Build history of the part. All positions in model axes, mm. Face numbers are marked on the shaded views. A direction names the side the tool comes from. Round coordinates to 2 decimals unless told otherwise and drop trailing zeros. Use one line per item in the form item = value. Start each with the question number.
Q1. 3-axis set-ups, long thin cutter, end or side, ignore diameter. For the marked faces 1 and 2: which of +Z, -Z, +X, -X, +Y, -Y reach the whole face in a straight line?
Q2. Saw through at A-A (y = -77.5). Count the separate pieces of the cut face and the enclosed holes in it, then the cut area to 3 significant figures.
Q3. Drill centre lines: line 1 (X direction, y = -75.5, z = -2); line 2 (Z direction, x = -5.5, y = 35.5); line 3 (X direction, y = -37.5, z = 6.5). Where is each one in solid material? Low to high.
Q4. Pin check, flat tips, straight feed: pin 1 (13.5 mm diameter, centred on x = -6, y = 66, fed in from +Z); pin 2 (0.5 mm diameter, centred on x = 22, y = -31.5, fed in from -Z); pin 3 (1.6 mm diameter, centred on x = 0.5, z = 8, fed in from -Y). Stop position of each tip, or through.
```python
from build123d import *

# Parameters (mm, degrees)
F2_DEPTH       = 250
F3_W           = 38
F3_H           = 13
F4_DEPTH       = 250
F5_R           = 9
F6_R           = 1
F7_T1_DEPTH    = 509.3674969976
F9_DEPTH       = 500.001
F12_DEPTH      = 13.5192964571
F12_DEPTH_BACK = 10.001
F13_T1_DEPTH   = 2
F13_T6_DEPTH   = 16.7634354909
F13_S7_R       = 200
F13_T8_DEPTH   = 11
F13_T12_DEPTH  = 16.7632527384
F13_S13_R      = 200
F13_T14_DEPTH  = 11
F13_T15_DEPTH  = 29.2634354909
F13_T17_DEPTH  = 27
F13_T19_DEPTH  = 29.2632527384
F14_DEPTH      = 13.5192964571
F14_DEPTH_BACK = 10.001


# Not quite as in the source:
# - a fillet or chamfer that OpenCascade refuses, or shapes differently, is made with other operations: its cross-section is extruded or revolved along the edge and cut away or added


with BuildPart() as f2:
    # F0 (on Front) → F2 (new body, symmetric)
    with BuildSketch(Plane.XZ):
        with BuildLine():
            Line((-22.5004640741, 10), (-45.5824640741, 10))
            Line((-45.5824640741, 10), (-57.5, 0))
            Line((-57.5, 0), (-57.5, -4))
            Line((-57.5, -4), (-40.1794919243, -14))
            ThreePointArc((-40.1794919243, -14), (0.0006744682, -9.9223168214), (40.1808408606, -14))
            Line((40.1808408606, -14), (57.5, -4.0007788087))
            Line((57.5, -4.0007788087), (57.5, -0.0007788087))
            Line((57.5, -0.0007788087), (45.5815359259, 10))
            Line((45.5815359259, 10), (22.4995359259, 10))
            Line((22.4995359259, 10), (22.4995359259, 8.7))
            Line((22.4995359259, 8.7), (-22.5004640741, 8.7))
            Line((-22.5004640741, 8.7), (-22.5004640741, 10))
        make_face()
    extrude(amount=F2_DEPTH, both=True)

    # F3 (on Front) → F4 (cut, symmetric)
    with BuildSketch(Plane.XZ):
        with Locations((0, 0.2)):
            Rectangle(F3_W, F3_H)
    extrude(amount=F4_DEPTH, both=True, mode=Mode.SUBTRACT)

    # F5
    f5_edges = [f2.edges().sort_by_distance(p)[0] for p in [
        (45.581536, 0, 10),
        (40.180841, 0, -14),
        (-45.582464, 0, 10),
        (-40.179492, 0, -14),
    ]]
    fillet(f5_edges, radius=F5_R)

    # F6
    f6_edges = [f2.edges().sort_by_distance(p)[0] for p in [
        (57.5, 0, -0.000779),
        (57.5, 0, -4.000779),
        (-57.5, 0, 0),
        (-57.5, 0, -4),
    ]]
    fillet(f6_edges, radius=F6_R)

    # F7: fillet of radius 2 on 2 edges, made by hand

    # F7_s2 → F7_t1 (cut)
    with BuildSketch(Plane.XZ.offset(-254.6837484988)):
        with BuildLine():
            ThreePointArc((24.3730353255, 10), (23.2328599004, 9.6431676725), (22.4995359259, 8.7))
            Line((22.4995359259, 8.7), (22.4995359259, 10))
            Line((22.4995359259, 10), (24.3730353255, 10))
        make_face()
        with BuildLine():
            ThreePointArc((-22.5004640741, 8.7), (-23.2337880485, 9.6431676725), (-24.3739634736, 10))
            Line((-24.3739634736, 10), (-22.5004640741, 10))
            Line((-22.5004640741, 10), (-22.5004640741, 8.7))
        make_face()
    extrude(amount=F7_T1_DEPTH, mode=Mode.SUBTRACT)

    # F8 (on face) → F9 (cut, through all)
    with BuildSketch(Plane.XZ.offset(250)):
        with BuildLine():
            Line((-21, -9.0169369236), (-21, 6.6999997944))
            Line((-21, 6.6999997944), (-22.5004640741, 6.6999997944))
            ThreePointArc((-22.5004640741, 6.6999997944), (-23.2337879899, 7.6431676078), (-24.3739634736, 8))
            Line((-24.3739634736, 8), (-42.3067319657, 8))
            ThreePointArc((-42.3067319657, 8), (-44.7008729689, 7.5778483455), (-46.8062452335, 6.3623111018))
            Line((-46.8062452335, 6.3623111018), (-55.5, -0.9326153163))
            Line((-55.5, -0.9326153163), (-55.5, -2.8452994616))
            Line((-55.5, -2.8452994616), (-42.102284203, -10.5804742836))
            ThreePointArc((-42.102284203, -10.5804742836), (-39.7790708711, -11.4186713119), (-37.3093621422, -11.3978569477))
            ThreePointArc((-37.3093621422, -11.3978569477), (-29.178975147, -10.0409819041), (-21, -9.0169369236))
        make_face()
        with BuildLine():
            Line((22.5004640741, 6.6999997944), (21, 6.6999997944))
            Line((21, 6.6999997944), (21, -9.0169369236))
            ThreePointArc((21, -9.0169369236), (29.178975147, -10.0409819041), (37.3093621422, -11.3978569477))
            ThreePointArc((37.3093621422, -11.3978569477), (39.7790708711, -11.4186713119), (42.102284203, -10.5804742836))
            Line((42.102284203, -10.5804742836), (55.5, -2.8452994616))
            Line((55.5, -2.8452994616), (55.5, -0.9326153163))
            Line((55.5, -0.9326153163), (46.8062452335, 6.3623111018))
            ThreePointArc((46.8062452335, 6.3623111018), (44.7008729689, 7.5778483455), (42.3067319657, 8))
            Line((42.3067319657, 8), (24.3739634736, 8))
            ThreePointArc((24.3739634736, 8), (23.2337879899, 7.6431676078), (22.5004640741, 6.6999997944))
        make_face()
    extrude(amount=-F9_DEPTH, mode=Mode.SUBTRACT)

    # F11 (on Top) → F12 (cut, two sides)
    with BuildSketch(Plane.XY) as f12_sk:
        Polygon((-68.0004640741, -346), (67.9995359259, -346), (67.9995359259, -216), (43.2970899738, -250), (15.9995359259, -250), (15.9995359259, -140), (-16.0004640741, -140), (-16.0004640741, -250), (-43.2980181219, -250), (-68.0004640741, -216), align=None)
    extrude(amount=-F12_DEPTH, mode=Mode.SUBTRACT)
    extrude(f12_sk.sketch, amount=F12_DEPTH_BACK, mode=Mode.SUBTRACT)

    # F13: fillet of radius 5 on 8 edges, made by hand

    # F13_s2 → F13_t1 (join)
    with BuildSketch(Plane.XY.offset(6.7)):
        with BuildLine():
            ThreePointArc((-11.0004640741, -140), (-14.53599798, -141.4644660941), (-16.0004640741, -145))
            Line((-16.0004640741, -145), (-16.0004640741, -140))
            Line((-16.0004640741, -140), (-11.0004640741, -140))
        make_face()
        with BuildLine():
            ThreePointArc((15.9995359259, -145), (14.5350698319, -141.4644660941), (10.9995359259, -140))
            Line((10.9995359259, -140), (15.9995359259, -140))
            Line((15.9995359259, -140), (15.9995359259, -145))
        make_face()
    extrude(amount=F13_T1_DEPTH)


with BuildPart() as f13_tool4:
    # F13_s5 → F13_t6 (new body)
    with BuildSketch(Plane.XY.offset(-23.0634354909)):
        with BuildLine():
            ThreePointArc((-16.0004640741, -145), (-14.53599798, -141.4644660941), (-11.0004640741, -140))
            Line((-11.0004640741, -140), (-16.0004640741, -140))
            Line((-16.0004640741, -140), (-16.0004640741, -145))
        make_face()
    extrude(amount=F13_T6_DEPTH)

    # F13_s7 → F13_t8 (cut, symmetric)
    with BuildSketch(Plane.XZ.offset(142.5)):
        with Locations((0.0006744682, -209.9223168214)):
            Circle(F13_S7_R)
    extrude(amount=F13_T8_DEPTH, both=True, mode=Mode.SUBTRACT)


with BuildPart() as f2_1:
    add(f2.part)

    # F13_t3: union F13_tool4
    add(f13_tool4.part)


with BuildPart() as f13_tool10:
    # F13_s11 → F13_t12 (new body)
    with BuildSketch(Plane.XY.offset(-23.0632527384)):
        with BuildLine():
            ThreePointArc((15.9995359259, -145), (14.5350698319, -141.4644660941), (10.9995359259, -140))
            Line((10.9995359259, -140), (15.9995359259, -140))
            Line((15.9995359259, -140), (15.9995359259, -145))
        make_face()
    extrude(amount=F13_T12_DEPTH)

    # F13_s13 → F13_t14 (cut, symmetric)
    with BuildSketch(Plane.XZ.offset(142.5)):
        with Locations((0.0006744682, -209.9223168214)):
            Circle(F13_S13_R)
    extrude(amount=F13_T14_DEPTH, both=True, mode=Mode.SUBTRACT)


with BuildPart() as f2_2:
    add(f2_1.part)

    # F13_t9: union F13_tool10
    add(f13_tool10.part)

    # F13_s16 → F13_t15 (cut)
    with BuildSketch(Plane.XY.offset(-23.0634354909)):
        with BuildLine():
            ThreePointArc((-21.0004640741, -250), (-17.4649301681, -248.5355339059), (-16.0004640741, -245))
            Line((-16.0004640741, -245), (-16.0004640741, -250))
            Line((-16.0004640741, -250), (-21.0004640741, -250))
        make_face()
    extrude(amount=F13_T15_DEPTH, mode=Mode.SUBTRACT)

    # F13_s18 → F13_t17 (cut)
    with BuildSketch(Plane.XY.offset(-5.8)):
        with BuildLine():
            ThreePointArc((20.9995359259, -250), (17.46400202, -248.5355339059), (15.9995359259, -245))
            Line((15.9995359259, -245), (15.9995359259, -250))
            Line((15.9995359259, -250), (20.9995359259, -250))
        make_face()
        with BuildLine():
            ThreePointArc((-16.0004640741, -245), (-17.4649301681, -248.5355339059), (-21.0004640741, -250))
            Line((-21.0004640741, -250), (-16.0004640741, -250))
            Line((-16.0004640741, -250), (-16.0004640741, -245))
        make_face()
    extrude(amount=F13_T17_DEPTH, mode=Mode.SUBTRACT)

    # F13_s20 → F13_t19 (cut)
    with BuildSketch(Plane.XY.offset(-23.0632527384)):
        with BuildLine():
            ThreePointArc((20.9995359259, -250), (17.46400202, -248.5355339059), (15.9995359259, -245))
            Line((15.9995359259, -245), (15.9995359259, -250))
            Line((15.9995359259, -250), (20.9995359259, -250))
        make_face()
    extrude(amount=F13_T19_DEPTH, mode=Mode.SUBTRACT)

    # F10 (on Top) → F14 (cut, two sides)
    with BuildSketch(Plane.XY) as f14_sk:
        with BuildLine():
            ThreePointArc((-57.5, 200), (0, 257.5), (57.5, 200))
            Line((57.5, 200), (57.5, 280))
            Line((57.5, 280), (-57.5, 280))
            Line((-57.5, 280), (-57.5, 200))
        make_face()
    extrude(amount=-F14_DEPTH, mode=Mode.SUBTRACT)
    extrude(f14_sk.sketch, amount=F14_DEPTH_BACK, mode=Mode.SUBTRACT)


solid = f2_2.part
```
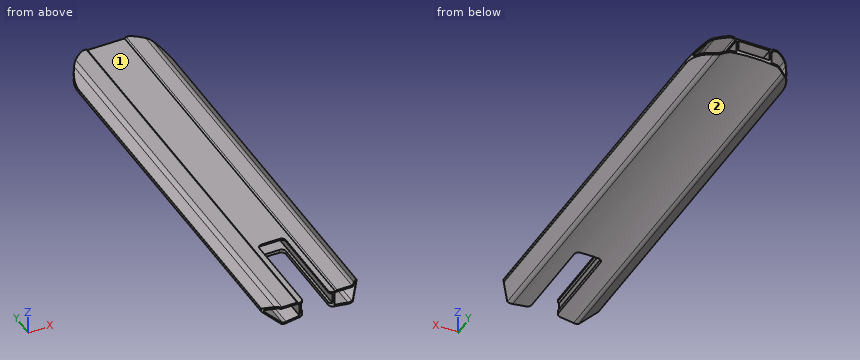
Report:
q1.face_1 = +Z, +Y, -Y
q1.face_2 = -Z, +Y, -Y
q2.separate_pieces = 1
q2.enclosed_holes = 3
q2.area = 622 mm²
q3.line_1 = -57.5 to -55.5, -21 to -19, 19 to 21, 55.5 to 57.5
q3.line_2 = -10 to -6.3, 6.7 to 8.7
q3.line_3 = -49.75 to -46.64, -21 to -19, 19 to 21, 46.64 to 49.75
q4.pin_1 = 8.7
q4.pin_2 = -11.16
q4.pin_3 = -140
